Verification items for the finished model (mm, model axes). A direction names the side the tool comes from. Coordinates: 2 decimals unless noted, no trailing zeros. Write each loop counter-clockwise with the first axis right and the second up, starting at its lowest first coordinate (ties: lowest second). Pieces come first, ordered by that corner, then holes. Notation, with made-up numbers: (82, 25) -> (89, 25) arc R24 ccw to (89, 53) -> close; hole circle Ø6 at (-33, -10). An arc over 180 degrees is marked (long way). Use CSV: the item, a comma, the result in double quotes.
```python
from build123d import *

# Parameters (mm, degrees)
SKETCH1_R           = 15
SKETCH1_R_2         = 10
BOSS_EXTRUDE1_DEPTH = 30
BOSS_EXTRUDE2_DEPTH = 5


with BuildPart() as part:
    # Sketch1 → Boss-Extrude1 (new body)
    with BuildSketch(Plane.XY):
        Circle(SKETCH1_R)
        Circle(SKETCH1_R_2, mode=Mode.SUBTRACT)
    extrude(amount=-BOSS_EXTRUDE1_DEPTH)

    # Sketch2 → Boss-Extrude2 (add, symmetric)
    with BuildSketch(Plane.XY.offset(-15)):
        with BuildLine():
            Line((-40, 15), (0, 15))
            ThreePointArc((0, 15), (-15, 0), (0, -15))
            Line((0, -15), (-40, -15))
            ThreePointArc((-40, -15), (-55, 0), (-40, 15))
        make_face()
        with BuildLine():
            Line((-40, 7.5), (-25, 7.5))
            ThreePointArc((-25, 7.5), (-17.5, 0), (-25, -7.5))
            Line((-25, -7.5), (-40, -7.5))
            ThreePointArc((-40, -7.5), (-47.5, 0), (-40, 7.5))
        make_face(mode=Mode.SUBTRACT)
    extrude(amount=BOSS_EXTRUDE2_DEPTH, both=True)


solid = part.part
```
1) Cross-section at A-A (x = -35). Record the boundary of the cut face in (y, z), plus the area to 3 significant figures.
Return value:
outline,"(-15, -20) -> (-7.5, -20) -> (-7.5, -10) -> (-15, -10) -> close; (7.5, -20) -> (15, -20) -> (15, -10) -> (7.5, -10) -> close"
area,"150 mm2"
2) Mould release check, pull along X, two halves, no side actions. Record for faces 4 (the flat face through (-33, 10, -20)), 5 (the cylindrical face through (-55, 0, -15)), 6 (the cylindrical face through (-2.17, -9.76, -14.79)): released by +X, released by -X, zero draft, split by the parting line, or undercut.
Return value:
face 4,"zero draft"
face 5,"released by -X"
face 6,"undercut"
3) Cross-section at D-D (x = -12). Record the boundary of the cut face in (y, z), plus the area to 3 significant figures.
Return value:
outline,"(-15, -20) -> (-9, -20) -> (-9, -30) -> (9, -30) -> (9, -20) -> (15, -20) -> (15, -10) -> (9, -10) -> (9, 0) -> (-9, 0) -> (-9, -10) -> (-15, -10) -> close"
area,"660 mm2"
4) Cross-section at C-C (y = -9). Record the boundary of the cut face in (x, z).
Return value:
outline,"(-52, -20) -> (-12, -20) -> (-12, -30) -> (-4.36, -30) -> (-4.36, 0) -> (-12, 0) -> (-12, -10) -> (-52, -10) -> close; (4.36, -30) -> (12, -30) -> (12, 0) -> (4.36, 0) -> close"
5) Gauge pin test, flat ends, axial feed: pin 1 (8 mm diameter, centred on y = 7.5, z = -22.5, fed in from +X); pin 2 (5 mm diameter, centred on y = -3, z = -14.5, fed in from +X); pin 3 (1.5 mm diameter, centred on x = -45.5, z = -19, fed in from +Y). Record the tip position at first contact, or that the pin passes through.
Return value:
pin 1,"x = 14.59"
pin 2,"x = 14.99"
pin 3,"y = 14.23"
6) Scan lines: L1, parallel to X at y = -3.5, z = -17.5; L2, parallel to Y at x = 0, z = -17; L3, parallel to Y at x = -39.5, z = -14.5. Record each from-to range of solid material in increasing order.
Return value:
L1,"-54.59 to -46.63, -18.37 to -9.37, 9.37 to 14.59"
L2,"-15 to -10, 10 to 15"
L3,"-15 to -7.5, 7.5 to 15"
7) Cross-section at B-B (y = 0). Record the boundary of the cut face in (x, z).
Return value:
outline,"(-55, -20) -> (-47.5, -20) -> (-47.5, -10) -> (-55, -10) -> close; (-17.5, -20) -> (-15, -20) -> (-15, -30) -> (-10, -30) -> (-10, 0) -> (-15, 0) -> (-15, -10) -> (-17.5, -10) -> close; (10, -30) -> (15, -30) -> (15, 0) -> (10, 0) -> close"
8) Set-up check for faces 1 (the cylindrical face through (-47.5, -0.16, -14.93)), 2 (the flat face through (-33, 10, -10)), 3 (the cylindrical face through (14.307, 4.506, -14.79)): record each of +Z, -Z, +X, -X, +Y, -Y from which the full face is reachable in a straight line by a thin tool's end or side.
Return value:
face 1,"+Z, -Z"
face 2,"+Z, -X"
face 3,"none"
